Autodesk Inventor part; units mm, degrees
ref_plane "YZ Plane" through (0, 0, 0) normal (1, 0, 0) x (0, 1, 0)
ref_plane "XZ Plane" through (0, 0, 0) normal (0, 1, 0) x (-1, 0, 0)
ref_plane "XY Plane" through (0, 0, 0) normal (0, 0, 1) x (1, 0, 0)
sketch "Boceto1" plane through (0, 0, 0) normal (0, 0, 1) x (1, 0, 0)
  arc A0 (-303.9864, -15.0738) -> (-301.0136, -44.9262) centre (-302.5, -30) ccw
  arc A1 (301.4864, 15.0738) -> (298.5136, 44.9262) centre (300, 30) ccw
  line L0 (-303.9864, -15.0738) -> (298.5136, 44.9262)
  line L1 (301.4864, 15.0738) -> (-301.0136, -44.9262)
  line L2 (-361.4241, -13.7591) -> (297.8199, 51.8917)
  arc A2 (302.1801, 8.1083) -> (297.8199, 51.8917) centre (300, 30) ccw
  line L3 (302.1801, 8.1083) -> (-300.3199, -51.8917)
  arc A3 (-304.6801, -8.1083) -> (-300.3199, -51.8917) centre (-302.5, -30) ccw
  point P0 (0, 0)
  dimension "d0" = 30
  dimension "d1" = 30
  dimension "d2" = 300
  dimension "d3" = 302.5
  dimension "d4" = 30
  dimension "d5" = 30
  dimension "d6" = 7
  dimension "d8" = 7
extrude "Extrusión1" add sketch "Boceto1" along normal blind 10
properties part number "faja"
Here's how the part is built. I have some questions about the finished solid (model axes, mm). A direction names the side the tool comes from. Give positions to 0.01 mm unless a question says otherwise; leave off trailing zeros. Order: outer loops, then holes, each group sorted by start corner. A loop starts at its lowest first (then second) coordinate and runs counter-clockwise, first axis right, second up. Notation, with made-up numbers: (62.5, 25) -> (66.5, 25) arc R29 ccw to (66.5, 50) -> close; hole circle Ø9 at (35, -34). An arc over 180 degrees is marked (long way). Use a Markdown table: item, result. Add a question column.
Item 1: I need wall thicknesses on line 1 (Y direction, x = 47, z = 7); line 2 (Y direction, x = 43.5, z = 0.5). Which ranges of each line are inside material? Lowest first, please.
Item 2: Will these pins go through, and if not, where does the flat tip stop? pin 1 (6 mm diameter, centred on x = 4.5, z = 3.5, fed in from +Y); pin 2 (6 mm diameter, centred on x = 199.5, z = 1.5, fed in from -Y); pin 3 (1.5 mm diameter, centred on x = 195, z = 3.5, fed in from -Y); pin 4 (2 mm diameter, centred on x = -154.5, y = 4, fed in from -Z).
Item 3: For faces 1 (the face through (-3, 16, 0)), 2 (the face through (-317.39, -31.81, 4.93)), which set-ups out of +Z, -Z, +X, -X, +Y, -Y let a thin tool reach every point of the face, with its end or its side?
Item 4: Imagine slicing it at C-C on x = 58. Please give me the cut outline in (y, z).
Item 5: Imagine slicing it at A-A on y = 37. Please give me the cut outline in (x, z), plus the area to 3 significant figures.
Item 6: If we mould it in two halves opening along X, with no side actions, what happens to faces 3 (the face through (5.15, -21.47, 4.93)), 4 (the face through (-3, 16, 10)), 5 (the face through (4.5, -14.5, 4.9)), 6 (the face through (-7.65, 21.47, 4.93))? For each: pulls with the +X half, pulls with the -X half, needs draft (parallel to the pull), parting line crosses it, or undercut.
Item 7: Imagine slicing it at B-B on z = 7. Please give me the cut outline in (x, y).
Data:
| question | item | result |
|---|---|---|
| 1 | line 1 | y = -17.3 to -10.27, 19.88 to 26.91 |
| 1 | line 2 | y = -17.65 to -10.62, 19.53 to 26.57 |
| 2 | pin 1 | stops at y = 22.98 |
| 2 | pin 2 | stops at y = -2.42 |
| 2 | pin 3 | stops at y = -2.64 |
| 2 | pin 4 | stops at z = 0 |
| 3 | face 1 | -Z, +X, -X, +Y, -Y |
| 3 | face 2 | +Z, -Z |
| 4 | outline | (-16.21, 0) -> (-9.17, 0) -> (-9.17, 10) -> (-16.21, 10) -> close; (20.97, 0) -> (28.01, 0) -> (28.01, 10) -> (20.97, 10) -> close |
| 5 | outline | (148.28, 0) -> (218.92, 0) -> (218.92, 10) -> (148.28, 10) -> close; (313.27, 0) -> (320.86, 0) -> (320.86, 10) -> (313.27, 10) -> close |
| 5 | area | 782 mm² |
| 6 | face 3 | pulls with the +X half |
| 6 | face 4 | needs draft |
| 6 | face 5 | undercut |
| 6 | face 6 | pulls with the -X half |
| 7 | outline | (-304.68, -8.11) arc R22 ccw to (-300.32, -51.89) -> (302.18, 8.11) arc R22 ccw to (297.82, 51.89) -> close; hole (-303.99, -15.07) arc R15 ccw to (-301.01, -44.93) -> (301.49, 15.07) arc R15 ccw to (298.51, 44.93) -> close |
